from build123d import *

# Parameters (mm, degrees)
CYLINDER103_R               = 2.2
CYLINDER103_DEPTH           = 30
CYLINDER099_R               = 2.2
CYLINDER099_DEPTH           = 100
ARRAY001_Z_COUNT            = 4
ARRAY001_Z_PITCH            = 15
BOX048_W                    = 3
BOX048_H                    = 10
BOX048_DEPTH                = 20
BOX_W                       = 3
BOX_H                       = 17
BOX_DEPTH                   = 27
ARRAY_X_COUNT               = 2
ARRAY_X_PITCH               = 44
CYLINDER097_R               = 8
CYLINDER097_DEPTH           = 20
CYLINDER097_PLACEMENT_ANGLE = 10
BOX047_W                    = 47
BOX047_H                    = 5.6
BOX047_DEPTH                = 20
CYLINDER096_W               = 11.5
CYLINDER096_H               = 20
CYLINDER096_ANGLE           = 160
CYLINDER096_PLACEMENT_ANGLE = 10
FILLET_R                    = 2


with BuildPart() as insert_hole:
    # Cylinder103 → Cylinder103 (new body)
    with BuildSketch(Plane(origin=(15, -19, 10), x_dir=(1, 0, 0), z_dir=(0, 1, 0))):
        Circle(CYLINDER103_R)
    extrude(amount=CYLINDER103_DEPTH)


with BuildPart() as m3_bolt_insert_fusion001:
    # Part__Mirroring007: instance of insert hole
    add(insert_hole.part.mirror(Plane(origin=(0, 0, 0), x_dir=(0, -1, 0), z_dir=(1, 0, 0))))

    # Fusion076: union insert hole
    add(insert_hole.part)


with BuildPart() as m4_hole_array:
    # Cylinder099 → Cylinder099 (new body)
    with BuildSketch(Plane(origin=(-50, 9, 6), x_dir=(0, 0, -1), z_dir=(1, 0, 0))):
        Circle(CYLINDER099_R)
    extrude(amount=CYLINDER099_DEPTH)

    # Array001 Z: m4 hole array ×4


with BuildPart() as m4_hole_array_1:
    add(m4_hole_array.part)
    with Locations(*[(0, 0, i * ARRAY001_Z_PITCH) for i in range(1, ARRAY001_Z_COUNT)]):
        add(m4_hole_array.part)


with BuildPart() as wall_cube001:
    # Box048 → Box048 (new body)
    with BuildSketch(Plane(origin=(0, -9, 0), x_dir=(1, 0, 0), z_dir=(0, 0, 1))):
        with Locations((1.5, 5)):
            Rectangle(BOX048_W, BOX048_H)
    extrude(amount=BOX048_DEPTH)


with BuildPart() as walls_with_holes:
    # Box → Box (new body)
    with BuildSketch(Plane.XY):
        with Locations((1.5, 8.5)):
            Rectangle(BOX_W, BOX_H)
    extrude(amount=BOX_DEPTH)

    # Fusion: union wall cube001
    add(wall_cube001.part)


with BuildPart() as walls_with_holes_1:
    # Fusion placement: moved
    add(walls_with_holes.part.moved(Location((-23.5, 0, 0))))

    # Array X: walls with holes ×2


with BuildPart() as walls_with_holes_2:
    add(walls_with_holes_1.part)
    with Locations(*[(i * ARRAY_X_PITCH, 0, 0) for i in range(1, ARRAY_X_COUNT)]):
        add(walls_with_holes_1.part)

    # Cut: cut m4 hole array
    add(m4_hole_array_1.part, mode=Mode.SUBTRACT)


with BuildPart() as walls_with_holes_3:
    # Cut placement: moved
    add(walls_with_holes_2.part.moved(Location((0, 10, 0))))


with BuildPart() as pile_extraction001:
    # Cylinder097 → Cylinder097 (new body)
    with BuildSketch(Plane.XY):
        Circle(CYLINDER097_R)
    extrude(amount=CYLINDER097_DEPTH)


with BuildPart() as pile_extraction001_1:
    # Cylinder097 placement: moved
    add(pile_extraction001.part.rotate(Axis((0, 0, 0), (0, 0, 1)), CYLINDER097_PLACEMENT_ANGLE))


with BuildPart() as cube004:
    # Box047 → Box047 (new body)
    with BuildSketch(Plane(origin=(-23.5, 1.2, 0), x_dir=(1, 0, 0), z_dir=(0, 0, 1))):
        with Locations((23.5, 2.8)):
            Rectangle(BOX047_W, BOX047_H)
    extrude(amount=BOX047_DEPTH)


with BuildPart() as solder_with_walls_fillet_clone:
    # Cylinder096 → Cylinder096 (revolve)
    with BuildSketch(Plane.XZ):
        with Locations((5.75, 10)):
            Rectangle(CYLINDER096_W, CYLINDER096_H)
    revolve(axis=Axis((0, 0, 0), (0, 0, 1)), revolution_arc=CYLINDER096_ANGLE)


with BuildPart() as solder_with_walls_fillet_clone_1:
    # Cylinder096 placement: moved
    add(solder_with_walls_fillet_clone.part.rotate(Axis((0, 0, 0), (0, 0, 1)), CYLINDER096_PLACEMENT_ANGLE))

    # Fusion072: union Cube004
    add(cube004.part)

    # Cut023016: cut pile extraction001
    add(pile_extraction001_1.part, mode=Mode.SUBTRACT)

    # Fusion073: union walls with holes
    add(walls_with_holes_3.part)

    # Cut023015: cut m3 bolt insert fusion001
    add(m3_bolt_insert_fusion001.part, mode=Mode.SUBTRACT)


with BuildPart() as solder_with_walls_fillet_clone_2:
    # Cut023015 placement: moved
    add(solder_with_walls_fillet_clone_1.part.moved(Location((0, -11, 0))))

    # Fillet
    fillet_edges = [solder_with_walls_fillet_clone_2.edges().sort_by_distance(p)[0] for p in [
        (-22, -1, 27),
        (-22, 16, 27),
        (-22, 16, 0),
        (22, -1, 27),
        (22, 16, 27),
        (22, 16, 0),
    ]]
    fillet(fillet_edges, radius=FILLET_R)


with BuildPart() as solder_with_walls_fillet_clone_3:
    # Body placement: moved
    add(solder_with_walls_fillet_clone_2.part.moved(Location((0, 0, 75))))


solid = solder_with_walls_fillet_clone_3.part
Geometry check sheet. Reference: the model listing, model coordinates, mm. A direction names the side the tool comes from. Round coordinates to 2 decimals unless told otherwise and drop trailing zeros. Order: outer loops, then holes, each group sorted by start corner. A loop starts at its lowest first (then second) coordinate and runs counter-clockwise, first axis right, second up. Notation, with made-up numbers: M -36,-27 L -1,-27 A19 ccw -1,-13 Z; hole C -31,-35 d10. An arc over 180 degrees is marked long. Answer in a Markdown table with one row per item. Add a question column.
Item 1: Sectioned sample at B-B, the plane y = 8. Enter the section's corners in (x, z), plus the area to 3 significant figures.
Item 2: Depth check by flat-ended pin: pin 1 Ø3.5 at (y, z) = (8, 96) entering from +X; pin 2 Ø5 at (x, z) = (-5, 90) entering from +Y (3 decimals); pin 3 Ø4 at (x, z) = (-14.5, 89) entering from -Y; pin 4 Ø8 at (x, z) = (-9.5, 79) entering from +Y. Enter the tip coordinate at first touch or a pass-through.
Item 3: Sectioned sample at C-C, the plane x = 15. Enter the section's corners in (y, z).
Item 4: Set-up check for faces 4 (the face through (-22, -1, 97)), 5 (the face through (20.5, 6, 88)), 6 (the face through (-22.02, 8.66, 93.9)), 7 (the face through (14.1, -9.8, 82.6)): record each of +Z, -Z, +X, -X, +Y, -Y from which the full face is reachable in a straight line by a thin tool's end or side.
Item 5: Sectioned sample at A-A, the plane z = 81. Enter the section's corners in (x, y).
Item 6: Material ranges on L1, parallel to Z at x = 22.65, y = 8; L2, parallel to Y at x = 21.7, z = 96; L3, parallel to X at y = 10.5, z = 85, recorded low to high. Write a range as [from, to].
Item 7: Draft check along Z on faces 1 (the face through (22.02, -0.43, 101.4)), 2 (the face through (21.98, 8.66, 78.9)), 3 (the face through (-15, -4.2, 82.6)). Enter one of: released by +Z, released by -Z, zero draft, split by the parting line, or undercut.
Item 8: Sectioned sample at D-D, the plane z = 96. Enter the section's corners in (x, y), plus the area to 3 significant figures.
Filled in:
| question | item | result |
|---|---|---|
| 1 | outline | M -23.5,75 L -20.5,75 L -20.5,78.8 L -23.5,78.8 Z; M -23.5,83.2 L -20.5,83.2 L -20.5,93.8 L -23.5,93.8 Z; M -23.5,98.2 L -20.5,98.2 L -20.5,102 L -23.5,102 Z; M 20.5,75 L 23.5,75 L 23.5,78.8 L 20.5,78.8 Z; M 20.5,83.2 L 23.5,83.2 L 23.5,93.8 L 20.5,93.8 Z; M 20.5,98.2 L 23.5,98.2 L 23.5,102 L 20.5,102 Z |
| 1 | area | 109 mm² |
| 2 | pin 1 | passes through |
| 2 | pin 2 | stops at y = 0.225 |
| 2 | pin 3 | stops at y = -9.8 |
| 2 | pin 4 | stops at y = -0.9 |
| 3 | outline | M -9.8,75 L -4.2,75 L -4.2,82.8 L -9.8,82.8 Z; M -9.8,87.2 L -4.2,87.2 L -4.2,95 L -9.8,95 Z |
| 4 | face 4 | +Z, +X, -X, -Y |
| 4 | face 5 | +Z, -Z, +Y |
| 4 | face 6 | +X, -X |
| 4 | face 7 | +Z, -Z, -Y |
| 5 | outline | M -23.5,-10 L -20.5,-10 L -20.5,-9.8 L -7.91,-9.8 A8 cw 7.91,-9.8 L 20.5,-9.8 L 20.5,-10 L 23.5,-10 L 23.5,5.8 L 20.5,5.8 L 20.5,-4.2 L 9.27,-4.2 A11.5 ccw -9.27,-4.2 L -20.5,-4.2 L -20.5,5.8 L -23.5,5.8 Z; M -23.5,10.2 L -20.5,10.2 L -20.5,16 L -23.5,16 Z; M 20.5,10.2 L 23.5,10.2 L 23.5,16 L 20.5,16 Z |
| 6 | L1 | z = [75, 78.8], [83.2, 93.8], [98.2, 102] |
| 6 | L2 | y = [-1, 5.8], [10.2, 16] |
| 6 | L3 | x = [-23.5, -20.5], [20.5, 23.5] |
| 7 | face 1 | released by +Z |
| 7 | face 2 | undercut |
| 7 | face 3 | zero draft |
| 8 | outline | M -23.5,-1 L -20.5,-1 L -20.5,5.8 L -23.5,5.8 Z; M -23.5,10.2 L -20.5,10.2 L -20.5,16 L -23.5,16 Z; M 20.5,-1 L 23.5,-1 L 23.5,5.8 L 20.5,5.8 Z; M 20.5,10.2 L 23.5,10.2 L 23.5,16 L 20.5,16 Z |
| 8 | area | 75.6 mm² |
